Source: three-view drawing plus pictorial views. Frame: mm from the lowest corner of the part. Give positions to 0.01 mm unless a question says otherwise; leave off trailing zeros. Loops run counter-clockwise (first coordinate to the right, second up) from the corner with the lowest first, then second, coordinate; pieces in that order, holes last. Notation, with made-up numbers: M 45,-3.5 L 86,-3.5 A13 cw 86,0.5 Z; hole C 89.5,62 d5. An arc over 180 degrees is marked long. Answer as a JSON object with one key per item and string values. Group by question number.
1) Section query D-D on z = 9. Return loops of the section in (x, y).
2) Ray query, L1, parallel to Y at x = 7.5, z = 3.75; L2, parallel to X at y = 4.5, z = 8.75; L3, parallel to Y at x = 10.75, z = 5.75. Return the intervals inside material, ascending.
3) Section query A-A on x = 7.5. Return loops of the section in (y, z).
4) Draft query along Y for the marked faces 1 and 2. Return one class per face: +Y half, -Y half, draft (parallel to the pull), parting line (faces both ways), or undercut.
5) First-contact query: P1, Ø5, axis at x = 4.5, z = 5, coming from the +Y side; P2, Ø4, axis at y = 6, z = 4.5, coming from the -X side; P3, Ø5, axis at x = 2.5, z = 9, coming from the +Y side; P4, Ø1.5, axis at x = 5, y = 2.5, coming from the -Z side. Flat tips, straight axial feed; report the tip coordinate or a pass-through.
6) Section query C-C on z = 3. Return loops of the section in (x, y), plus the area to 3 significant figures.
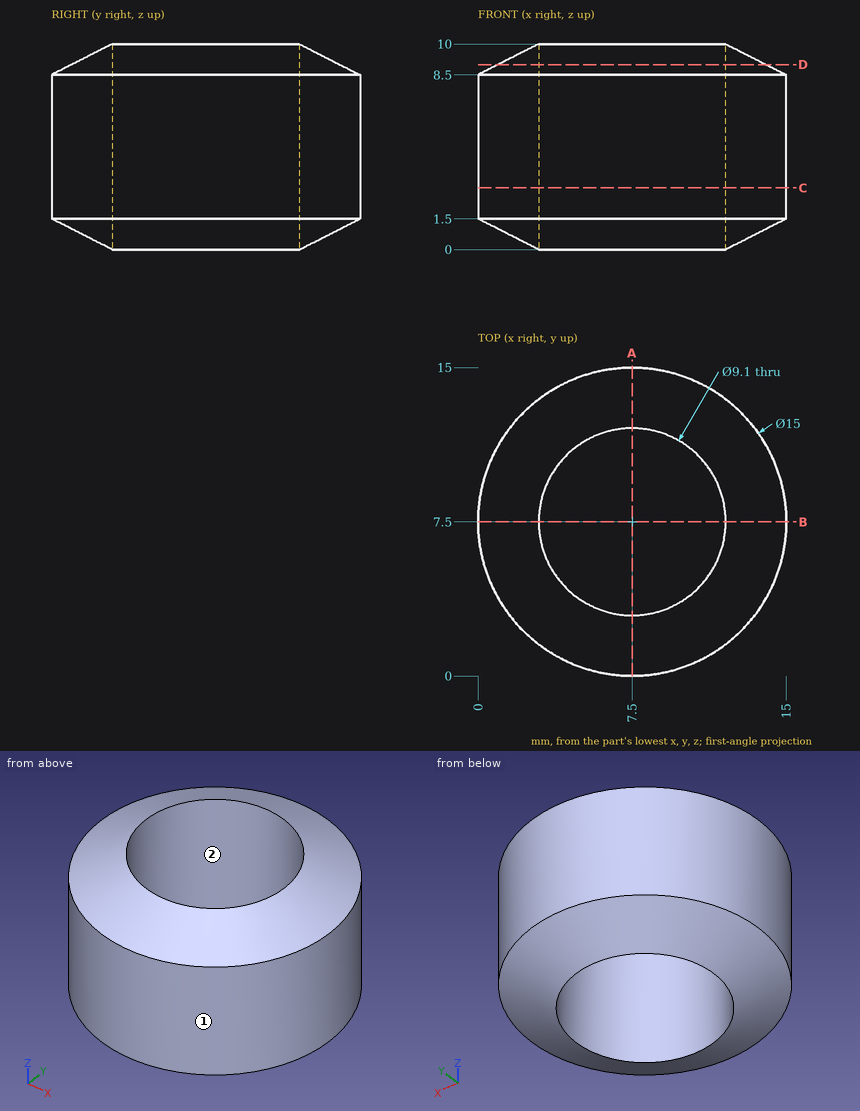
Output:
{
 "1": {"outline": "C 7.5,7.5 d13.03; hole C 7.5,7.5 d9.1"},
 "2": {"L1": "y = 0 to 2.95, 12.05 to 15", "L2": "x = 1.17 to 4.08, 10.92 to 13.83", "L3": "y = 0.74 to 4.32, 10.68 to 14.26"},
 "3": {"outline": "M 0,1.5 L 2.95,0 L 2.95,10 L 0,8.5 Z; M 12.05,0 L 15,1.5 L 15,8.5 L 12.05,10 Z"},
 "4": {"face 1": "parting line", "face 2": "undercut"},
 "5": {"P1": "stops at y = 14.98", "P2": "stops at x = 0", "P3": "stops at y = 14.55", "P4": "stops at z = 0.15"},
 "6": {"outline": "C 7.5,7.5 d15; hole C 7.5,7.5 d9.1", "area": "112 mm^2"}
}
